The model under review builds one solid part; all positions refer to its coordinate system, in mm. Face numbers are marked on the shaded views. Round coordinates to 2 decimals unless told otherwise and drop trailing zeros. Order: outer loops, then holes, each group sorted by start corner. A loop starts at its lowest first (then second) coordinate and runs counter-clockwise, first axis right, second up. Notation, with made-up numbers: (2.5, -25.5) -> (28.5, -25.5) arc R35 ccw to (28.5, 11.5) -> close; hole circle Ø6 at (-20.75, 6). An arc over 180 degrees is marked (long way). Return JSON: item names as keys, results as strings. Group by question number.
from build123d import *

# Parameters (mm, degrees)
SKETCH1_W           = 50.55571166
SKETCH1_H           = 25.842581666
SKETCH1_R           = 2.413
SKETCH1_R_2         = 2.249766629
SKETCH1_R_3         = 6.35
BOSS_EXTRUDE1_DEPTH = 3.175
FILLET1_R           = 2.54


with BuildPart() as part:
    # Sketch1 → Boss-Extrude1 (new body)
    with BuildSketch(Plane.XY):
        Rectangle(SKETCH1_W, SKETCH1_H)
        with Locations((-17.4625, 0)):
            Circle(SKETCH1_R, mode=Mode.SUBTRACT)
        with Locations((17.4625, 0)):
            Circle(SKETCH1_R_2, mode=Mode.SUBTRACT)
        Circle(SKETCH1_R_3, mode=Mode.SUBTRACT)
    extrude(amount=BOSS_EXTRUDE1_DEPTH)

    # Fillet1
    fillet1_edges = [part.edges().sort_by_distance(p)[0] for p in [
        (25.27785583, -12.921290833, 1.5875),
        (-25.27785583, -12.921290833, 1.5875),
        (-25.27785583, 12.921290833, 1.5875),
        (25.27785583, 12.921290833, 1.5875),
    ]]
    fillet(fillet1_edges, radius=FILLET1_R)


solid = part.part
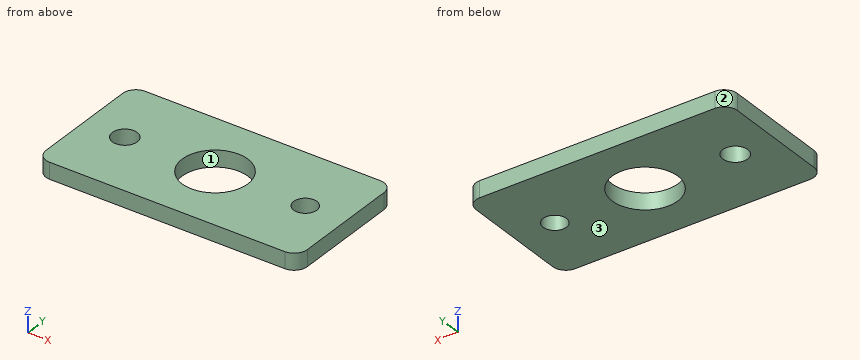
Item 1: Consider section A-A on x = 0. State the section outline as (y, z) points (3 decimals), plus the area to 3 significant figures.
Item 2: Wall thickness on line 1 along Y through (x, z) = (0, 1.3); line 2 along X through (y, z) = (0.5, 1.55); line 3 along X through (y, z) = (2.5, 0.8): over which ranges is each line inside the solid? List them lowest first.
Item 3: Consider section C-C on z = 2.6. State the section outline as (x, y) points.
Item 4: Consider section D-D on x = 17. State the section outline as (y, z) points (3 decimals), plus the area to 3 significant figures.
Item 5: The part is to be moulded in two halves that separate along X. For the marked faces 1, 2 and 3, say which applies: +X half, -X half, draft (parallel to the pull), parting line (faces both ways), or undercut.
Item 6: Consider section B-B on y = 0. Give the number of separate pieces and of enclosed holes in the cut face, plus the area to 3 significant figures.
Item 7: Insertion check: pin 1 Ø10 at (x, y) = (0, 0) entering from -Z. The pin has a flat end and moves straight along its axis. Give the tip position at first contact, or say it passes through.
Values:
{
 "1": {"outline": "(-12.921, 0) -> (-6.35, 0) -> (-6.35, 3.175) -> (-12.921, 3.175) -> close; (6.35, 0) -> (12.921, 0) -> (12.921, 3.175) -> (6.35, 3.175) -> close", "area": "41.7 mm^2"},
 "2": {"line 1": "-12.92 to -6.35, 6.35 to 12.92", "line 2": "-25.28 to -19.82, -15.1 to -6.33, 6.33 to 15.27, 19.66 to 25.28", "line 3": "-25.28 to -5.84, 5.84 to 25.28"},
 "3": {"outline": "(-25.28, -10.38) arc R2.54 ccw to (-22.74, -12.92) -> (22.74, -12.92) arc R2.54 ccw to (25.28, -10.38) -> (25.28, 10.38) arc R2.54 ccw to (22.74, 12.92) -> (-22.74, 12.92) arc R2.54 ccw to (-25.28, 10.38) -> close; hole circle Ø4.83 at (-17.46, 0); hole circle Ø12.7 at (0, 0); hole circle Ø4.5 at (17.46, 0)"},
 "4": {"outline": "(-12.921, 0) -> (-2.202, 0) -> (-2.202, 3.175) -> (-12.921, 3.175) -> close; (2.202, 0) -> (12.921, 0) -> (12.921, 3.175) -> (2.202, 3.175) -> close", "area": "68.1 mm^2"},
 "5": {"face 1": "undercut", "face 2": "-X half", "face 3": "draft"},
 "6": {"separate pieces": "4", "enclosed holes": "0", "area": "90.6 mm^2"},
 "7": {"pin 1": "through"}
}
